Could you check a few things on this model? Use its own coordinates, in mm. A direction names the side the tool comes from. Give positions to 0.01 mm unless a question says otherwise; leave off trailing zeros. Write each loop counter-clockwise with the first axis right and the second up, starting at its lowest first coordinate (ties: lowest second). Pieces come first, ordered by that corner, then holes. Notation, with made-up numbers: M -17.75,-8.5 L -2.75,-8.5 A21 ccw -2.75,2.5 Z; hole C 51,-19 d10. An arc over 180 degrees is marked long. Write each question's results on one line, items separated by ' | '. Start each with the question number.
Autodesk Inventor part; units mm, degrees
ref_plane "YZ Plane" through (0, 0, 0) normal (1, 0, 0) x (0, 1, 0)
ref_plane "XZ Plane" through (0, 0, 0) normal (0, 1, 0) x (-1, 0, 0)
ref_plane "XY Plane" through (0, 0, 0) normal (0, 0, 1) x (1, 0, 0)
sketch "スケッチ1" plane through (0, 0, 0) normal (0, 0, 1) x (1, 0, 0)
  circle A0 centre (0, 0) radius 73.5 construction
  line L0 (-90, -170) -> (90, -170)
  line L1 (90, -170) -> (90, 70)
  line L2 (90, 70) -> (-90, 70)
  line L3 (-90, 70) -> (-90, -170)
  line L4 (-90, -170) -> (90, 70) construction
  line L5 (90, -170) -> (-90, 70) construction
  point P0 (0, -50)
  point P1 (0, -50)
  dimension "d25" = 147
  dimension "d26" = 240
  dimension "d71" = 180
  dimension "d76" = 70
extrude "押し出し2" add sketch "スケッチ1" along normal mid plane 8
sketch "スケッチ5" plane through (0, 0, 4) normal (0, 0, 1) x (1, 0, 0)
  line L0 (-50.5, -113.75) -> (85, -113.75)
  line L1 (85, -113.75) -> (85, -70.25)
  line L2 (85, -70.25) -> (-50.5, -70.25)
  line L3 (-50.5, -70.25) -> (-50.5, -113.75)
  line L4 (-50.5, -113.75) -> (85, -70.25) construction
  line L5 (85, -113.75) -> (-50.5, -70.25) construction
  line L6 (90, -170) -> (90, 70)
  point P0 (0, 0)
  point P1 (17.25, -92)
  point P2 (17.25, -92)
  dimension "d40" = 135.5
  dimension "d41" = 43.5
  dimension "d73" = 92
  dimension "d74" = 5
hole "穴3" at (-50.5, -70.25, 4) at (-50.5, -113.75, 4) at (85, -113.75, 4) at (85, -70.25, 4) direction (0, 0, -1) diameter 2.459 depth 8.8 tip angle 118
sketch "スケッチ6" plane through (0, 0, -4) normal (0, 0, -1) x (-1, 0, 0)
  circle A0 centre (0, 0) radius 30
  dimension "d54" = 60
extrude "押し出し3" cut sketch "スケッチ6" against normal through all
fillet "フィレット3" radius 10 4 edges at (90, 70, 0) (-90, 70, 0) (90, -170, 0) (-90, -170, 0)
sketch "スケッチ7" plane through (0, 0, 4) normal (0, 0, 1) x (1, 0, 0)
  line L0 (-25, -68) -> (42, -68)
  line L1 (42, -68) -> (42, -152)
  line L2 (42, -152) -> (-25, -152)
  line L3 (-25, -152) -> (-25, -68)
  line L4 (-25, -68) -> (42, -152) construction
  line L5 (42, -68) -> (-25, -152) construction
  line L6 (-80, -170) -> (80, -170)
  line L7 (-90, 60) -> (-90, -160)
  line L8 (90, -160) -> (90, 60)
  point P0 (0, 0)
  point P1 (8.5, -110)
  dimension "d59" = 67
  dimension "d60" = 84
  dimension "d70" = 110
  dimension "d75" = 48
hole "穴4" at (-25, -152, 4) at (-25, -68, 4) at (42, -68, 4) at (42, -152, 4) direction (0, 0, -1) diameter 2.459 depth 8.8 tip angle 118
sketch "スケッチ8" plane through (0, 0, -4) normal (0, 0, -1) x (-1, 0, 0)
  arc A0 (-80, 70) -> (-90, 60) centre (-80, 60) ccw
  arc A1 (90, 60) -> (80, 70) centre (80, 60) ccw
  arc A2 (80, -170) -> (90, -160) centre (80, -160) ccw
  arc A3 (-90, -160) -> (-80, -170) centre (-80, -160) ccw
  point P0 (0, 0)
hole "穴5" at (80, -160, -4) at (-80, -160, -4) at (-80, 60, -4) at (80, 60, -4) direction (0, 0, 1) diameter 3.2 end through all counterbore diameter 6.5 counterbore depth 3
sketch "スケッチ9" plane through (0, 0, 4) normal (0, 0, 1) x (1, 0, 0)
  line L0 (-80, -170) -> (80, -170)
  line L1 (80, 70) -> (-80, 70)
  point P0 (0, 0)
  point P1 (-60, -144)
  point P2 (60, -144)
  point P3 (-60, 44)
  point P4 (60, 44)
  dimension "d84" = 60
  dimension "d85" = 60
  dimension "d86" = 26
  dimension "d94" = 26
hole "穴6" at (-60, -144, 4) at (60, -144, 4) at (-60, 44, 4) at (60, 44, 4) direction (0, 0, -1) diameter 4.134 end through all
sketch "スケッチ3" plane through (0, 0, -4) normal (0, 0, 1) x (1, 0, 0)
  circle A0 centre (0, 0) radius 62.5
  point P0 (-16.1762, 60.3704)
  point P1 (-44.1942, 44.1942)
  point P2 (-60.3704, 16.1762)
  point P3 (-60.3704, -16.1762)
  point P4 (-44.1942, -44.1942)
  point P5 (-16.1762, -60.3704)
  point P6 (16.1762, -60.3704)
  point P7 (44.1942, -44.1942)
  point P8 (60.3704, -16.1762)
  point P9 (60.3704, 16.1762)
  point P10 (44.1942, 44.1942)
  point P11 (16.1762, 60.3704)
  dimension "d8" = 125
  dimension "d11" = 360
  dimension "d20" = 0
hole "穴1" at (-16.1762, 60.3704, -4) at (-44.1942, 44.1942, -4) at (-60.3704, 16.1762, -4) at (-60.3704, -16.1762, -4) at (-44.1942, -44.1942, -4) at (-16.1762, -60.3704, -4) at (16.1762, -60.3704, -4) at (44.1942, -44.1942, -4) at (60.3704, -16.1762, -4) at (60.3704, 16.1762, -4) at (44.1942, 44.1942, -4) at (16.1762, 60.3704, -4) direction (0, 0, 1) diameter 4.3 end through all counterbore diameter 8 counterbore depth 4
sketch "スケッチ4" plane through (0, 0, 4) normal (0, 0, 1) x (1, 0, 0)
  line L0 (-80, -150) -> (80, -150)
  line L1 (80, -150) -> (80, 50)
  line L2 (80, 50) -> (-80, 50)
  line L3 (-80, 50) -> (-80, -150)
  line L4 (-80, -150) -> (80, 50) construction
  line L5 (80, -150) -> (-80, 50) construction
  line L6 (90, 70) -> (-90, 70)
  line L7 (-90, -170) -> (90, -170)
  line L8 (79.8007, -110) -> (-79.8007, -110)
  line L9 (-79.8007, -110) -> (-79.8007, 10)
  line L10 (-79.8007, 10) -> (79.8007, 10)
  line L11 (79.8007, 10) -> (79.8007, -110)
  line L12 (79.8007, -110) -> (-79.8007, 10) construction
  line L13 (-79.8007, -110) -> (79.8007, 10) construction
  line L14 (40, -150) -> (-40, -150)
  line L15 (-40, -150) -> (-40, 50)
  line L16 (-40, 50) -> (40, 50)
  line L17 (40, 50) -> (40, -150)
  line L18 (40, -150) -> (-40, 50) construction
  line L19 (-40, -150) -> (40, 50) construction
  line L20 (79.6443, -70) -> (-79.6443, -70)
  line L21 (-79.6443, -70) -> (-79.6443, -30)
  line L22 (-79.6443, -30) -> (79.6443, -30)
  line L23 (79.6443, -30) -> (79.6443, -70)
  line L24 (79.6443, -70) -> (-79.6443, -30) construction
  line L25 (-79.6443, -70) -> (79.6443, -30) construction
  line L26 (0, 50) -> (0, -150)
  point P0 (0, 0)
  point P1 (0, -50)
  point P2 (0, -50)
  point P3 (60, 72.5)
  point P4 (-60, 72.5)
  point P5 (-90, 70)
  dimension "d30" = 160
  dimension "d31" = 200
  dimension "d72" = 20
  dimension "d96" = 40
  dimension "d97" = 40
  dimension "d98" = 40
hole "穴2" at (80, 50, 4) at (-80, 50, 4) at (-80, -150, 4) at (80, -150, 4) at (0, 50, 4) at (0, -150, 4) direction (0, 0, -1) diameter 4.134 end through all
sketch "スケッチ10" plane through (-90, -160, 4) normal (-1, 0, 0) x (0, 0, 1)
  line L0 (0, 230) -> (-8, 230)
  line L1 (-8, 0) -> (-8, 220)
  point P0 (-4, 160)
  point P1 (-4, 190)
  point P2 (-4, 110)
  point P3 (-4, 30)
  point P4 (-4, -50)
  point P5 (-4, -130)
  dimension "d99" = 40
  dimension "d102" = 80
  dimension "d107" = 4
hole "穴7" at (-90, 30, 0) at (-90, -50, 0) at (-90, -130, 0) at (-90, -210, 0) at (-90, -290, 0) direction (1, 0, 0) diameter 2.459 depth 8.8 tip angle 118
mirror "ミラー1" about plane through (0, 0, 0) normal (1, 0, 0) of "穴7"
equation "\"d82\" = Thickness"
equation "\"d18\" = Thickness"
equation "\"BendRadius\" = Thickness"
equation "\"BendReliefWidth\" = Thickness"
equation "\"BendReliefDepth\" = 0.5 * Thickness"
equation "\"CornerReliefSize\" = 4 * Thickness"
equation "\"MinimumRemnant\" = 2 * Thickness"
equation "\"TransitionRadius\" = BendRadius"
equation "\"JacobiRadiusSize\" = BendRadius"
equation "\"GapSize\" = Thickness"
equation "\"d2\" = Thickness"
properties part number "base5" material "鋼、炭素鋼"
Q1. I'm going to push flat-ended pins straight in: P1, Ø2, axis at y = 30, z = 0, coming from the +X side; P2, Ø2.5, axis at x = 60.5, y = 14.5, coming from the -Z side; P3, Ø3.5, axis at x = 0, y = -150, coming from the -Z side. Where does each tip first touch, or does it pass through?
Q2. Please list where these lines run through material, in increasing order: line 1 (Y direction, x = 0, z = 1); line 2 (X direction, y = -150, z = -2.5); line 3 (X direction, y = -113.75, z = 0.5). Write a range as [from, to].
Q3. If we section it at A-A (x = 8): Please give me the cut outline in (y, z).
Q4. If we section it at B-B (y = -9.5): Please give me the cut outline in (x, z), plus the area to 3 significant figures.
Q5. If we mould it in two halves opening along X, with no side actions, what happens to faces 1 (the face through (-1, -48, 4)), 2 (the face through (46, 46, 0)), 3 (the face through (-90, -48, 0))? For each: pulls with the +X half, pulls with the -X half, needs draft (parallel to the pull), parting line crosses it, or undercut.
Q6. For faces 4 (the face through (90, -52, 0)), 5 (the face through (63.92, -14.33, -1.97)), which set-ups out of +Z, -Z, +X, -X, +Y, -Y let a thin tool reach every point of the face, with its end or its side?
Determined:
1) P1: stops at x = 81.06 | P2: stops at z = 0 | P3: passes through
2) line 1: y = [-170, -152.07], [-147.93, -30], [30, 47.93], [52.07, 70] | line 2: x = [-90, -82.07], [-77.93, -2.07], [2.07, 77.93], [82.07, 90] | line 3: x = [-90, -51.73], [-49.27, 83.77], [86.23, 90]
3) outline: M -170,-4 L -28.91,-4 L -28.91,4 L -170,4 Z; M 28.91,-4 L 70,-4 L 70,4 L 28.91,4 Z
4) outline: M -90,-4 L -28.46,-4 L -28.46,4 L -90,4 Z; M 28.46,-4 L 90,-4 L 90,4 L 28.46,4 Z | area: 985 mm²
5) face 1: needs draft | face 2: undercut | face 3: pulls with the -X half
6) face 4: +Z, -Z, +X, +Y, -Y | face 5: -Z
